Study the drawing (mm; zero at the part's minimum x, y, z) and answer. A direction names the side the tool comes from. Give positions to 0.01 mm unless a question says otherwise; leave off trailing zeros. Order: outer loops, then holes, each group sorted by start corner. A loop starts at its lowest first (then second) coordinate and runs counter-clockwise, first axis right, second up.
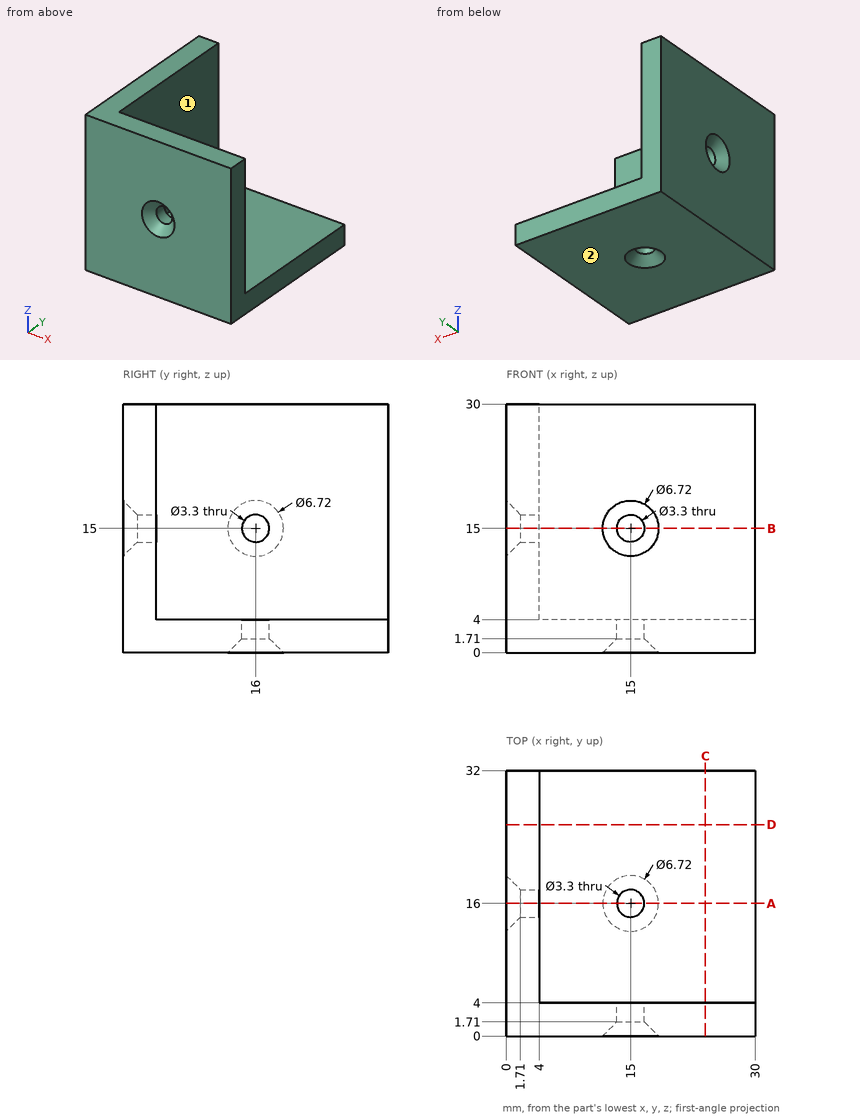
1) Find section A-A (y = 16). Write down the section's boundary in (x, z), then the cut area to 3 significant figures.
Geometry says:
outline: (0, 0) - (11.64, 0) - (13.35, 1.71) - (13.35, 4) - (4, 4) - (4, 13.35) - (1.71, 13.35) - (0, 11.64) - close; (0, 18.36) - (1.71, 16.65) - (4, 16.65) - (4, 30) - (0, 30) - close; (16.65, 1.71) - (18.36, 0) - (30, 0) - (30, 4) - (16.65, 4) - close
area: 192 mm2
2) Find section D-D (y = 25.5). Write down the section's boundary in (x, z), then the cut area to 3 significant figures.
Geometry says:
outline: (0, 0) - (30, 0) - (30, 4) - (4, 4) - (4, 30) - (0, 30) - close
area: 224 mm2
3) Given P1, Ø4, axis at y = 27, z = 23, coming from the +X side; P2, Ø12, axis at x = 24.5, y = 11.5, coming from the +Z side, each flat-ended and moving along its own axis, determine where each tip first touches the part or whether it passes through.
Geometry says:
P1: stops at x = 4
P2: stops at z = 4
4) Straight lines are drawn through the part: probe 1 along X at (y, z) = (3.3, 15); probe 2 along Z at (x, y) = (9.5, 8). For each, find the intervals that lie inside material, in ascending order.
Geometry says:
probe 1: x = 0 to 13.35, 16.65 to 30
probe 2: z = 0 to 4
5) Find section B-B (z = 15). Write down the section's boundary in (x, y).
Geometry says:
outline: (0, 0) - (11.64, 0) - (13.35, 1.71) - (13.35, 4) - (4, 4) - (4, 14.35) - (1.71, 14.35) - (0, 12.64) - close; (0, 19.36) - (1.71, 17.65) - (4, 17.65) - (4, 32) - (0, 32) - close; (16.65, 1.71) - (18.36, 0) - (30, 0) - (30, 4) - (16.65, 4) - close
6) Find section C-C (x = 24). Write down the section's boundary in (y, z).
Geometry says:
outline: (0, 0) - (32, 0) - (32, 4) - (4, 4) - (4, 30) - (0, 30) - close
7) A tool of negligible diameter and unlimited length cuts with its end or side. For the marked faces 1 and 2, from which of +Z, -Z, +X, -X, +Y, -Y can it reach the whole face along a straight path? Write none if from no direction.
Geometry says:
face 1: +Z, +X, +Y
face 2: -Z, +X, -X, +Y, -Y
